Read the model definition and answer for the solid it produces. Units are mm, in the model's axes. Face numbers are marked on the shaded views. Give positions to 0.01 mm unless a question says otherwise; leave off trailing zeros. Order: outer loops, then holes, each group sorted by start corner. A loop starts at its lowest first (then second) coordinate and runs counter-clockwise, first axis right, second up. Notation, with made-up numbers: (71.5, 47.25) - (75.5, 47.25) arc R32 ccw to (75.5, 80.25) - close; hole circle Ø7 at (63, -27). An arc over 180 degrees is marked (long way). Write item = value, one per line.
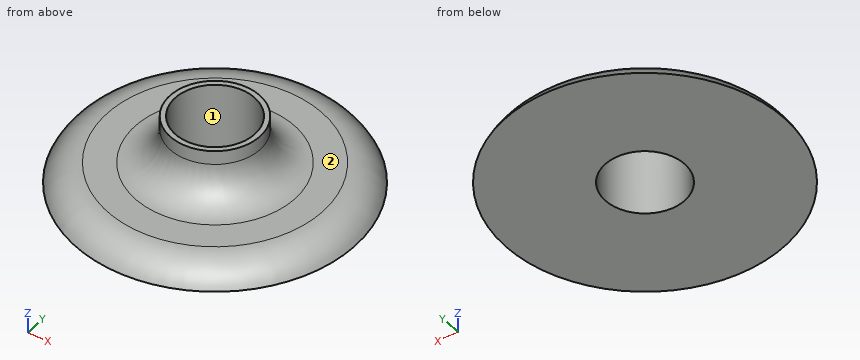
```python
from build123d import *

# Parameters (mm, degrees)
SKETCH1_R           = 50.8
BOSS_EXTRUDE1_DEPTH = 25.4
SKETCH2_R           = 14.478
CUT_EXTRUDE1_DEPTH  = 25.4
SKETCH3_OUTSIDE_W   = 132.782
SKETCH3_OUTSIDE_H   = 132.782
SKETCH3_OUTSIDE_R   = 16.333066569
CUT_EXTRUDE2_DEPTH  = 17.78
FILLET1_R           = 12.7
FILLET2_R           = 12.7


with BuildPart() as part:
    # Sketch1 → Boss-Extrude1 (new body)
    with BuildSketch(Plane.XY):
        with Locations((-23.323029636, 24.13527445)):
            Circle(SKETCH1_R)
    extrude(amount=BOSS_EXTRUDE1_DEPTH)

    # Sketch2 → Cut-Extrude1 (cut)
    with BuildSketch(Plane.XY.offset(25.4)):
        with Locations((-23.323029636, 24.13527445)):
            Circle(SKETCH2_R)
    extrude(amount=-CUT_EXTRUDE1_DEPTH, mode=Mode.SUBTRACT)

    # Sketch3 outside → Cut-Extrude2 (cut)
    with BuildSketch(Plane.XY.offset(25.4)):
        with Locations((-23.323, 24.135)):
            Rectangle(SKETCH3_OUTSIDE_W, SKETCH3_OUTSIDE_H)
        with Locations((-23.323029636, 24.13527445)):
            Circle(SKETCH3_OUTSIDE_R, mode=Mode.SUBTRACT)
    extrude(amount=-CUT_EXTRUDE2_DEPTH, mode=Mode.SUBTRACT)

    # Fillet1
    fillet1_edges = [part.edges().sort_by_distance(p)[0] for p in [
        (-39.656096206, 24.13527445, 7.62),
    ]]
    fillet(fillet1_edges, radius=FILLET1_R)

    # Fillet2
    # the kernel refuses this fillet: 12.7 mm, written as the material it takes off along each edge
    with BuildSketch(Plane(origin=(-23.323029636, 24.13527445, 7.62), x_dir=(1, 0, 0), z_dir=(0, 1, 0))) as fillet2_piece_1:
        with BuildLine():
            CenterArc((39.160257735, 12.7), FILLET2_R, 270, 66.421821522)
            Line((50.8, 7.62), (51.032794845, 7.5184))
            ThreePointArc((51.032794845, 7.5184), (51.054, 3.81), (51.054, 0))
            Line((51.054, 0), (50.8, -0.254))
            Line((50.8, -0.254), (39.160257735, -0.254))
            Line((39.160257735, -0.254), (39.160257735, 0))
        make_face()
    revolve(axis=Axis((-23.323029636, 24.13527445, 7.62), (0, 0, -1)), mode=Mode.SUBTRACT)


solid = part.part
```
1. Straight lines are drawn through the part: L1, parallel to X at y = 31, z = 23.5; L2, parallel to X at y = 37, z = 17.25; L3, parallel to Z at x = -31.5, y = -12. For each, find the intervals that lie inside material, in ascending order. Write a range as [from, to].
Recorded:
L1 = [-38.14, -36.07], [-10.58, -8.5]
L2 = [-33.99, -29.96], [-16.68, -12.66]
L3 = [0, 7.62]
2. Section A-A (z = 17) is taken. Determine the outline of the cut face in (x, y), and give its area (3 significant figures).
Recorded:
outline = circle Ø33.55 at (-23.32, 24.14); hole circle Ø28.96 at (-23.32, 24.14)
area = 225 mm^2
3. Flat-ended cylindrical pins translate along their axes: pin 1 (1.5 mm diameter, centred on x = -4.5, z = 5.5, fed in from +Y); pin 2 (5 mm diameter, centred on y = 16.5, z = 5, fed in from -X); pin 3 (6 mm diameter, centred on y = 39, z = 17, fed in from +X); pin 4 (17.5 mm diameter, centred on x = -23.32, y = 24.14, fed in from -Z). Find the tip coordinate at first contact, or state that the pin passes through.
Recorded:
pin_1 = 67.47
pin_2 = -72.12
pin_3 = -11.15
pin_4 = through
4. Determine the mould class of the marked faces 1 and 2 for opening direction X: +X half, -X half, draft (parallel to the pull), parting line (faces both ways), or undercut.
Recorded:
face_1 = undercut
face_2 = draft
5. Section B-B (z = 9.25) is taken. Determine the outline of the cut face in (x, y).
Recorded:
outline = circle Ø45.62 at (-23.32, 24.14); hole circle Ø28.96 at (-23.32, 24.14)
